```python
from build123d import *

# Parameters (mm, degrees)
F0_R     = 11.176
F1_DEPTH = 5.715


with BuildPart() as f1:
    # F0 (on Top) → F1 (new body)
    with BuildSketch(Plane.XY):
        with BuildLine():
            Line((14.771742, -20.371711), (14.771742, 0.583289))
            ThreePointArc((14.771742, 0.583289), (-1.103258, -15.291711), (-16.978258, 0.583289))
            Line((-16.978258, 0.583289), (-16.978258, -41.326711))
            Line((-16.978258, -41.326711), (14.771742, -41.326711))
            Line((14.771742, -41.326711), (14.771742, -20.371711))
        make_face()
        with Locations((-1.35877, -27.66218)):
            Circle(F0_R, mode=Mode.SUBTRACT)
        with BuildLine():
            ThreePointArc((-16.978258, 0.583289), (-1.103258, -15.291711), (14.771742, 0.583289))
            ThreePointArc((14.771742, 0.583289), (-1.103258, 16.458289), (-16.978258, 0.583289))
        make_face()
        with Locations((-1.103258, 0.583289)):
            Circle(F0_R, mode=Mode.SUBTRACT)
        with BuildLine():
            ThreePointArc((-16.978258, 0.583289), (-1.103258, 16.458289), (14.771742, 0.583289))
            Line((14.771742, 0.583289), (14.771742, 42.493289))
            Line((14.771742, 42.493289), (-16.978258, 42.493289))
            Line((-16.978258, 42.493289), (-16.978258, 21.538289))
            Line((-16.978258, 21.538289), (-16.978258, 0.583289))
        make_face()
        with Locations((-0.603735, 28.776065)):
            Circle(F0_R, mode=Mode.SUBTRACT)
        Polygon((40.171742, -20.371711), (14.771742, -20.371711), (14.771742, -41.326711), align=None)
        Polygon((-42.378258, 21.538289), (-16.978258, 21.538289), (-16.978258, 42.493289), align=None)
    extrude(amount=F1_DEPTH)


solid = f1.part
```
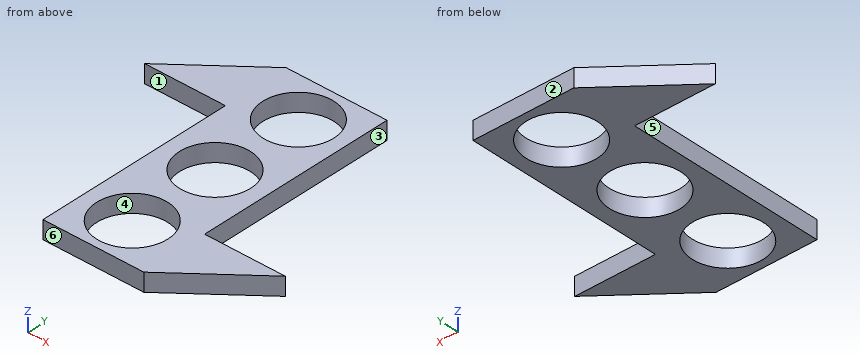
Check sheet for the modelled part. Datum: model origin and axes. Units: mm. Face numbers are marked on the shaded views. A direction names the side the tool comes from. Give positions to 0.01 mm unless a question says otherwise; leave off trailing zeros. Write each loop counter-clockwise with the first axis right and the second up, starting at its lowest first coordinate (ties: lowest second). Pieces come first, ordered by that corner, then holes.
Item 1: Cross-section at A-A (y = -22). Enter the section's corners in (x, z) (3 decimals), and give its area (3 significant figures).
Item 2: Cross-section at B-B (x = -3). Enter the section's corners in (y, z) (3 decimals).
Item 3: Cross-section at C-C (z = 1.55). Enter the section's corners in (x, y), and give its area (3 significant figures).
Item 4: Access from +Z, -Z, +X, -X, +Y, -Y to the whole of each face (thin tool, end or side, straight path). Record for the marked faces 1, 2 and 3.
Item 5: Draft check along X on the marked faces 4, 5 and 6. Enter one of: released by +X, released by -X, zero draft, split by the parting line, or undercut.
Item 6: Cross-section at D-D (y = 9.5). Enter the section's corners in (x, z) (3 decimals).
Item 7: Gauge pin test, flat ends, axial feed: pin 1 (1.7 mm diameter, centred on y = -7, z = 3, fed in from -X); pin 2 (3 mm diameter, centred on x = 26, z = 2.5, fed in from +Y); pin 3 (3 mm diameter, centred on x = -27, z = 2.5, fed in from -Y). Record the tip position at first contact, or that the pin passes through.
Item 8: Scan lines: L1, parallel to Y at x = 1, z = 5.1; L2, parallel to Y at x = -5, z = 0.5; L3, parallel to X at y = -13.5, z = 4.1. Record each from-to range of solid material in increasing order.
Report:
1. outline: (-16.978, 0) - (-10.994, 0) - (-10.994, 5.715) - (-16.978, 5.715) - close; (8.277, 0) - (38.198, 0) - (38.198, 5.715) - (8.277, 5.715) - close
1. area: 205 mm2
2. outline: (-41.327, 0) - (-38.717, 0) - (-38.717, 5.715) - (-41.327, 5.715) - close; (-16.607, 0) - (-10.431, 0) - (-10.431, 5.715) - (-16.607, 5.715) - close; (11.597, 0) - (17.86, 0) - (17.86, 5.715) - (11.597, 5.715) - close; (39.692, 0) - (42.493, 0) - (42.493, 5.715) - (39.692, 5.715) - close
3. outline: (-42.38, 21.54) - (-16.98, 21.54) - (-16.98, -41.33) - (14.77, -41.33) - (40.17, -20.37) - (14.77, -20.37) - (14.77, 42.49) - (-16.98, 42.49) - close; hole circle Ø22.35 at (-1.36, -27.66); hole circle Ø22.35 at (-1.1, 0.58); hole circle Ø22.35 at (-0.6, 28.78)
3. area: 2,020 mm2
4. face 1: +Z, -Z, -X, -Y
4. face 2: +Z, -Z, +X, -X, +Y
4. face 3: +Z, -Z, +X, +Y
5. face 4: undercut
5. face 5: released by -X
5. face 6: zero draft
6. outline: (-16.978, 0) - (-7.841, 0) - (-7.841, 5.715) - (-16.978, 5.715) - close; (5.634, 0) - (14.772, 0) - (14.772, 5.715) - (5.634, 5.715) - close
7. pin 1: stops at x = -16.98
7. pin 2: stops at y = -20.37
7. pin 3: stops at y = 21.54
8. L1: y = -41.33 to -38.59, -16.74 to -10.39, 11.56 to 17.72, 39.84 to 42.49
8. L2: y = -41.33 to -38.23, -17.1 to -9.89, 11.06 to 18.5, 39.05 to 42.49
8. L3: x = -16.98 to 14.77
